The listing builds one solid part. Answer for the finished solid, in the listing's coordinates (mm). A direction names the side the tool comes from. Round coordinates to 2 decimals unless told otherwise and drop trailing zeros. Loops run counter-clockwise (first coordinate to the right, second up) from the corner with the lowest first, then second, coordinate; pieces in that order, holes last. Notation, with made-up numbers: M 65.25,26.5 L 79.25,26.5 A21 cw 79.25,50.5 Z; hole C 78,-23.5 d4. An arc over 180 degrees is marked long. Answer as a JSON object with one key per item and string values.
```python
from build123d import *

# Parameters (mm, degrees)
SKETCH1_R           = 0.59563
BOSS_EXTRUDE1_DEPTH = 1.5875
FILLET1_R           = 0.762


with BuildPart() as part:
    # Sketch1 → Boss-Extrude1 (new body)
    with BuildSketch(Plane(origin=(0, 0, 0), x_dir=(1, 0, 0), z_dir=(0, 1, 0))):
        Polygon((0, 25), (4, 25), (6, 25), (6, 0), (4, 0), (0, 0), (0, 4), (4, 4), (4, 21), (0, 21), align=None)
        with Locations((2, 23)):
            Circle(SKETCH1_R, mode=Mode.SUBTRACT)
        with Locations((2, 2)):
            Circle(SKETCH1_R, mode=Mode.SUBTRACT)
    extrude(amount=BOSS_EXTRUDE1_DEPTH)

    # Fillet1
    fillet1_edges = [part.edges().sort_by_distance(p)[0] for p in [
        (6, 0.79375, -25),
        (6, 0.79375, 0),
        (0, 0.79375, 0),
        (0, 0.79375, -4),
        (0, 0.79375, -21),
        (0, 0.79375, -25),
    ]]
    fillet(fillet1_edges, radius=FILLET1_R)


solid = part.part
```
Item 1: A flat-ended cylindrical pin translates along its axis: P1, Ø1.5, axis at x = 2, z = -12, coming from the -Y side. Find the tip coordinate at first contact, or state that the pin passes through.
Values follow:
{"P1": "through"}
Item 2: Straight lines are drawn through the part: line 1 (Z direction, x = 2, y = 0.4); line 2 (X direction, y = 0.45, z = -2); line 3 (Z direction, x = 2.35, y = 1). For each, find the intervals that lie inside material, in ascending order.
Values follow:
{"line 1": "-25 to -23.6, -22.4 to -21, -4 to -2.6, -1.4 to 0", "line 2": "0 to 1.4, 2.6 to 6", "line 3": "-25 to -23.48, -22.52 to -21, -4 to -2.48, -1.52 to 0"}
Item 3: The part is cut by section C-C (x = 2). Give the vertices of the cut face in (y, z).
Values follow:
{"outline": "M 0,-25 L 1.59,-25 L 1.59,-23.6 L 0,-23.6 Z; M 0,-22.4 L 1.59,-22.4 L 1.59,-21 L 0,-21 Z; M 0,-4 L 1.59,-4 L 1.59,-2.6 L 0,-2.6 Z; M 0,-1.4 L 1.59,-1.4 L 1.59,0 L 0,0 Z"}
Item 4: Determine the mould class of faces 3 (the face through (4, 1, -12)), 4 (the face through (2, 1, -21)), 5 (the face through (1.87, 0.78, -22.42)) for opening direction X: released by +X, released by -X, zero draft, split by the parting line, or undercut.
Values follow:
{"face 3": "released by -X", "face 4": "zero draft", "face 5": "undercut"}
Item 5: The part is cut by section D-D (z = -19.25). Give the vertices of the cut face in (x, y), then the cut area to 4 significant figures.
Values follow:
{"outline": "M 4,0 L 6,0 L 6,1.59 L 4,1.59 Z", "area": "3.175 mm^2"}
Item 6: Which of the six approach directions +Z, -Z, +X, -X, +Y, -Y give full straight-line access (tool end or side, diameter ignored) to faces 1 (the face through (3, 1, -25)), 2 (the face through (2, 1, -4))?
Values follow:
{"face 1": "-Z, +X, -X, +Y, -Y", "face 2": "-X, +Y, -Y"}
Item 7: The part is cut by section A-A (z = -2). Give the vertices of the cut face in (x, y).
Values follow:
{"outline": "M 0,0 L 1.4,0 L 1.4,1.59 L 0,1.59 Z; M 2.6,0 L 6,0 L 6,1.59 L 2.6,1.59 Z"}
Item 8: The part is cut by section B-B (y = 0.3). Give the vertices of the cut face in (x, z), then the cut area to 3 significant figures.
Values follow:
{"outline": "M 0,-24.24 A0.76 ccw 0.76,-25 L 5.24,-25 A0.76 ccw 6,-24.24 L 6,-0.76 A0.76 ccw 5.24,0 L 0.76,0 A0.76 ccw 0,-0.76 L 0,-3.24 A0.76 ccw 0.76,-4 L 4,-4 L 4,-21 L 0.76,-21 A0.76 ccw 0,-21.76 Z; hole C 2,-23 d1.19; hole C 2,-2 d1.19", "area": "79.0 mm^2"}
